The drawing under review shows one solid part. Ordinate dimensions are in mm from its lowest x, y, z. Give positions to 0.01 mm unless a question says otherwise; leave off trailing zeros. Order: outer loops, then holes, each group sorted by start corner. A loop starts at its lowest first (then second) coordinate and runs counter-clockwise, first axis right, second up. Notation, with made-up numbers: (2.5, 81) -> (11.5, 81) arc R9 cw to (11.5, 91) -> close; hole circle Ø6 at (-3.5, 65). An arc over 180 degrees is marked (long way). Use a Markdown table: item, result. Add a question column.
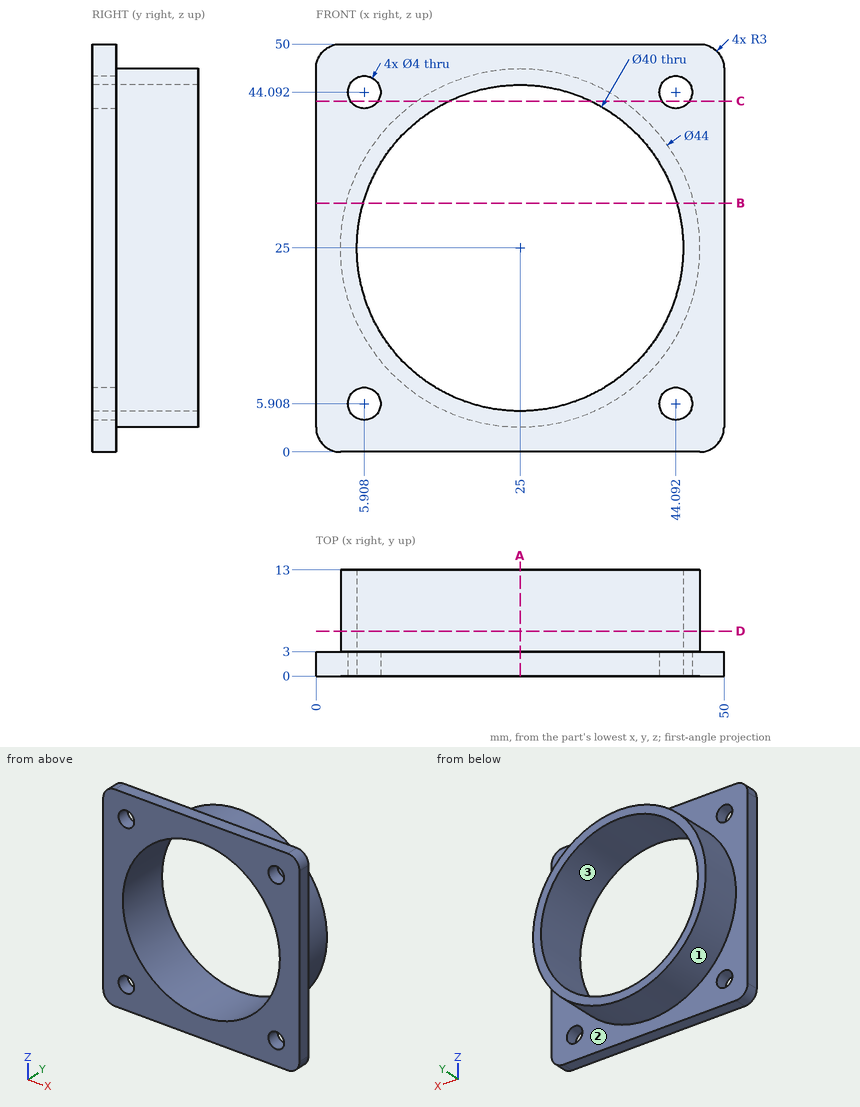
1) For L1, parallel to Z at x = 36, y = 2.5; L2, parallel to Y at x = 34, z = 3; L3, parallel to Z at x = 34.5, y = 0.5, list the stretches that pass through material, from the lowest coordinate up. Write a range as [from, to].
2) Add section A-A (x = 25). Give the boundary of the cut face in (y, z), then the cut area to 3 significant figures.
3) Insertion check: pin 1 (1 mm diameter, centred on x = 44, y = 10.5, fed in from -Z); pin 2 (6 mm diameter, centred on x = 14.5, y = 9, fed in from -Z); pin 3 (6.5 mm diameter, centred on x = 44.09, z = 44.09, fed in from +Y). Each pin has a flat end and moves straight along its axis. Give the tip position at first contact, or say it passes through.
4) Add section D-D (y = 5.5). Give the boundary of the cut face in (x, z), then the cut area to 3 significant figures.
5) Add section B-B (z = 30.5). Give the boundary of the cut face in (x, y), then the cut area to 3 significant figures.
6) Add section C-C (z = 43). Give the boundary of the cut face in (x, y), then the cut area to 3 significant figures.
7) The part is to be moulded in two halves that separate along Z. For the marked faces 1, 2 and 3, say which applies: +Z half, -Z half, draft (parallel to the pull), parting line (faces both ways), or undercut.
Worked answers:
| question | item | result |
|---|---|---|
| 1 | L1 | [0, 8.3], [41.7, 50] |
| 1 | L2 | [0, 3] |
| 1 | L3 | [0, 7.4], [42.6, 50] |
| 2 | outline | (0, 0) -> (3, 0) -> (3, 3) -> (13, 3) -> (13, 5) -> (0, 5) -> close; (0, 45) -> (13, 45) -> (13, 47) -> (3, 47) -> (3, 50) -> (0, 50) -> close |
| 2 | area | 70.0 mm^2 |
| 3 | pin 1 | z = 13.09 |
| 3 | pin 2 | z = 4.32 |
| 3 | pin 3 | y = 3 |
| 4 | outline | circle Ø44 at (25, 25); hole circle Ø40 at (25, 25) |
| 4 | area | 264 mm^2 |
| 5 | outline | (0, 0) -> (5.77, 0) -> (5.77, 13) -> (3.7, 13) -> (3.7, 3) -> (0, 3) -> close; (44.23, 0) -> (50, 0) -> (50, 3) -> (46.3, 3) -> (46.3, 13) -> (44.23, 13) -> close |
| 5 | area | 76.1 mm^2 |
| 6 | outline | (0, 0) -> (4.23, 0) -> (4.23, 3) -> (0, 3) -> close; (7.58, 0) -> (16.28, 0) -> (16.28, 13) -> (12.35, 13) -> (12.35, 3) -> (7.58, 3) -> close; (33.72, 0) -> (42.42, 0) -> (42.42, 3) -> (37.65, 3) -> (37.65, 13) -> (33.72, 13) -> close; (45.77, 0) -> (50, 0) -> (50, 3) -> (45.77, 3) -> close |
| 6 | area | 156 mm^2 |
| 7 | face 1 | parting line |
| 7 | face 2 | draft |
| 7 | face 3 | undercut |
